```python
from build123d import *

# Parameters (mm, degrees)
BOSS_EXTRUDE1_DEPTH              = 3
F_4_6_4_6_DIAMETER_HOLE1_D       = 4.6
CBORE_FOR_M6_5_SHSS1_D           = 7.2
CBORE_FOR_M6_5_SHSS1_CBORE_D     = 10
CBORE_FOR_M6_5_SHSS1_CBORE_DEPTH = 2
M10X1_0_TAPPED_HOLE1_D           = 5.1
F_3_0MM_DOWEL_HOLE1_D            = 3.4
F_5_0MM_DOWEL_HOLE1_D            = 5.5
FILLET3_R                        = 10


with BuildPart() as part:
    # Sketch1 → Boss-Extrude1 (new body)
    with BuildSketch(Plane(origin=(0, 6, 0), x_dir=(1, 0, 0), z_dir=(0, 1, 0))):
        Polygon((42, 42), (-42, 42), (-84, 42), (-84, -42), (-42, -42), (42, -42), align=None)
    extrude(amount=-BOSS_EXTRUDE1_DEPTH)

    # Ø4.6 (4.6) Diameter Hole1 (through all)
    with Locations(Plane(origin=(0, 3, 0), x_dir=(-1, 0, 0), z_dir=(0, -1, 0))):
        with Locations((0, 0)):
            Hole(F_4_6_4_6_DIAMETER_HOLE1_D / 2)

    # CBORE for M6.5 SHSS1 (through all)
    with Locations(Plane(origin=(0, 6, 0), x_dir=(1, 0, 0), z_dir=(0, 1, 0))):
        with Locations((29.85, 29.85), (29.85, -29.85)):
            CounterBoreHole(CBORE_FOR_M6_5_SHSS1_D / 2, CBORE_FOR_M6_5_SHSS1_CBORE_D / 2, CBORE_FOR_M6_5_SHSS1_CBORE_DEPTH)

    # M10x1.0 Tapped Hole1 (through all)
    with Locations(Plane(origin=(0, 6, 0), x_dir=(1, 0, 0), z_dir=(0, 1, 0))):
        with Locations((-29.85, -29.85), (-29.85, 29.85), (-29.85, 0)):
            Hole(M10X1_0_TAPPED_HOLE1_D / 2)

    # Ø3.0mm Dowel Hole1 (through all)
    with Locations(Plane(origin=(0, 6, 0), x_dir=(1, 0, 0), z_dir=(0, 1, 0))):
        with Locations((-75.5, 30.425), (-44.5, 30.425), (-44.5, -0.575), (-75.5, -0.575)):
            Hole(F_3_0MM_DOWEL_HOLE1_D / 2)

    # Ø5.0mm Dowel Hole1 (through all)
    with Locations(Plane(origin=(0, 6, 0), x_dir=(1, 0, 0), z_dir=(0, 1, 0))):
        with Locations((-60, 14.925)):
            Hole(F_5_0MM_DOWEL_HOLE1_D / 2)

    # Fillet3
    fillet3_edges = [part.edges().sort_by_distance(p)[0] for p in [
        (42, 4.5, -42),
        (42, 4.5, 42),
        (-84, 4.5, 42),
        (-84, 4.5, -42),
    ]]
    fillet(fillet3_edges, radius=FILLET3_R)


solid = part.part
```
CAD build for the part. Positions are in the model's coordinates, mm. A direction names the side the tool comes from. Coordinates: 2 decimals unless noted, no trailing zeros. Loops run counter-clockwise (first coordinate to the right, second up) from the corner with the lowest first, then second, coordinate; pieces in that order, holes last. Notation, with made-up numbers: (1, 8) - (30, 8) arc R23 cw to (30, 18) - close; hole circle Ø5 at (1.25, 39). An arc over 180 degrees is marked (long way). Return JSON: item names as keys, results as strings.
1. Probe L1, parallel to Z at x = 29.85, y = 5.15; L2, parallel to Z at x = -44.5, y = 4.4 (3 decimals); L3, parallel to Z at x = -29.85, y = 4.2. List the from-to ranges inside material, lowest first. Write a range as from..to.
Result:
{"L1": "z = -42..-34.85, -24.85..24.85, 34.85..42", "L2": "z = -42..-32.125, -28.725..-1.125, 2.275..42", "L3": "z = -42..-32.4, -27.3..-2.55, 2.55..27.3, 32.4..42"}
2. Band-saw the part on C-C (x = -44.5). Give the cut face in (y, z) (3 decimals), and give its area (3 significant figures).
Result:
{"outline": "(3, -42) - (6, -42) - (6, -32.125) - (3, -32.125) - close; (3, -28.725) - (6, -28.725) - (6, -1.125) - (3, -1.125) - close; (3, 2.275) - (6, 2.275) - (6, 42) - (3, 42) - close", "area": "232 mm2"}
3. Band-saw the part on D-D (y = 4.9). State how many separate pieces and enclosed holes the cut face has, and give its area (3 significant figures).
Result:
{"separate pieces": "1", "enclosed holes": "11", "area": "10,200 mm2"}
4. 3-axis set-ups, long thin cutter, end or side, ignore diameter. For faces 5 (the flat face through (26, 4, -31)), 6 (the flat face through (-84, 5, 0)): which of +Z, -Z, +X, -X, +Y, -Y reach the whole face in a straight line?
Result:
{"face 5": "+Y", "face 6": "+Z, -Z, -X, +Y, -Y"}
5. Band-saw the part on B-B (x = 0). Give the cut face in (y, z).
Result:
{"outline": "(3, -42) - (6, -42) - (6, -2.3) - (3, -2.3) - close; (3, 2.3) - (6, 2.3) - (6, 42) - (3, 42) - close"}
6. Mould opens along Z. For faces 1 (the flat face through (-22, 6, -1)), 2 (the cylindrical face through (-42.8, 4.5, 0.5)), 3 (the flat face through (26, 4, 29)), 4 (the flat face through (-20, 5, -42)) say: released by +Z, released by -Z, zero draft, split by the parting line, or undercut.
Result:
{"face 1": "zero draft", "face 2": "undercut", "face 3": "undercut", "face 4": "released by -Z"}
7. Band-saw the part on A-A (x = -29.85). Give the cut face in (y, z), and give its area (3 significant figures).
Result:
{"outline": "(3, -42) - (6, -42) - (6, -32.4) - (3, -32.4) - close; (3, -27.3) - (6, -27.3) - (6, -2.55) - (3, -2.55) - close; (3, 2.55) - (6, 2.55) - (6, 27.3) - (3, 27.3) - close; (3, 32.4) - (6, 32.4) - (6, 42) - (3, 42) - close", "area": "206 mm2"}
